```python
from build123d import *

# Parameters (mm, degrees)
ESQUISSE1_R             = 7
EXTRUSION1_DEPTH        = 100
ESQUISSE2_R             = 5
ESQUISSE2_R_2           = 2.5
EXTRUSION2_DEPTH        = 143
EXTRUSION2_DEPTH_BACK   = 36
ESQUISSE3_OUTSIDE_W     = 52.018
ESQUISSE3_OUTSIDE_H     = 52.018
ESQUISSE3_OUTSIDE_R     = 4.25
ENL_V_MAT_EXTRU_1_DEPTH = 3.5
ESQUISSE4_W             = 2
ESQUISSE4_H             = 3
ENL_V_MAT_EXTRU_2_DEPTH = 8
CHANFREIN1_SIZE         = 0.5


with BuildPart() as part:
    # Esquisse1 → Extrusion1 (new body)
    with BuildSketch(Plane(origin=(0, 0, 0), x_dir=(0, 0, -1), z_dir=(1, 0, 0))):
        Circle(ESQUISSE1_R)
    extrude(amount=EXTRUSION1_DEPTH)

    # Esquisse2 → Extrusion2 (add, two sides)
    with BuildSketch(Plane(origin=(0, 0, 0), x_dir=(0, 0, -1), z_dir=(1, 0, 0))) as extrusion2_sk:
        Circle(ESQUISSE2_R)
        Circle(ESQUISSE2_R_2, mode=Mode.SUBTRACT)
    extrude(amount=EXTRUSION2_DEPTH)
    extrude(extrusion2_sk.sketch, amount=-EXTRUSION2_DEPTH_BACK)

    # Esquisse3 outside → Enlèv. mat.-Extru.1 (cut)
    with BuildSketch(Plane.ZY.offset(36)):
        Rectangle(ESQUISSE3_OUTSIDE_W, ESQUISSE3_OUTSIDE_H)
        Circle(ESQUISSE3_OUTSIDE_R, mode=Mode.SUBTRACT)
    extrude(amount=-ENL_V_MAT_EXTRU_1_DEPTH, mode=Mode.SUBTRACT)

    # Esquisse4 → Enlèv. mat.-Extru.2 (cut, through all)
    with BuildSketch(Plane.XY):
        with Locations((-35, 0)):
            Rectangle(ESQUISSE4_W, ESQUISSE4_H)
    extrude(amount=ENL_V_MAT_EXTRU_2_DEPTH, mode=Mode.SUBTRACT)

    # Chanfrein1
    chanfrein1_edges = [part.edges().sort_by_distance(p)[0] for p in [
        (-36, 0, -4.25),
        (143, 0, 5),
    ]]
    chamfer(chanfrein1_edges, length=CHANFREIN1_SIZE)


solid = part.part
```
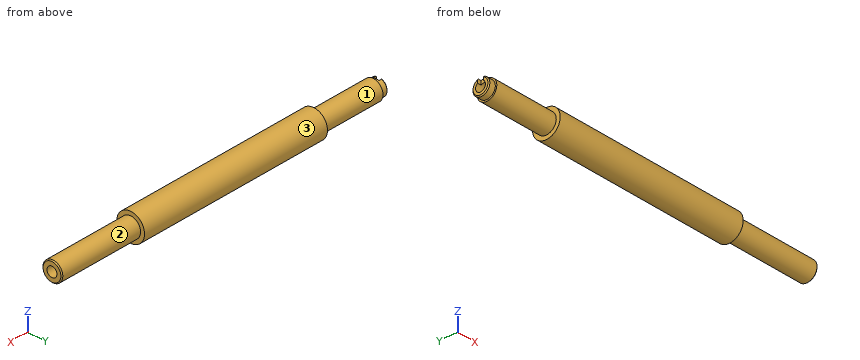
For this review, take the finished solid that the model builds, in its own axes (mm). Face numbers are marked on the shaded views. A direction names the side the tool comes from. Give positions to 0.01 mm unless a question says otherwise; leave off trailing zeros. Write each loop counter-clockwise with the first axis right and the second up, starting at its lowest first coordinate (ties: lowest second). Pieces come first, ordered by that corner, then holes.
Item 1: Wall thickness on probe 1 along Y at (x, z) = (-17.5, 0); probe 2 along X at (y, z) = (0.25, 2): over which ranges is each line inside the solid? List them lowest first.
Item 2: Take a section at B-B (z = 0). Give the boundary of the cut face in (x, y).
Item 3: Machinability: for the marked faces 1, 2 and 3, which of the approach directions +Z, -Z, +X, -X, +Y, -Y give a long, thin tool a straight path to every point of the face, cutting with its end or side? Answer none if there is none.
Item 4: Insertion check: P1, Ø5.5, axis at y = 1, z = -0.5, coming from the -X side; P2, Ø3, axis at x = 112, z = -1, coming from the -Y side; P3, Ø1, axis at x = 9, z = 5, coming from the -Y side; P4, Ø4, axis at x = 109, z = 4.5, coming from the -Y side. Each pin has a flat end and moves straight along its axis. Give the tip position at first contact, or say it passes through.
Item 5: Take a section at D-D (x = 60). Give the boundary of the cut face in (y, z).
Item 6: Take a section at A-A (y = 0). Give the boundary of the cut face in (x, z).
Item 7: Take a section at C-C (x = -16). Give the boundary of the cut face in (y, z).
Established:
1. probe 1: y = -5 to -2.5, 2.5 to 5
1. probe 2: x = 0 to 100
2. outline: (-36, -3.75) - (-35.5, -4.25) - (-32.5, -4.25) - (-32.5, -5) - (0, -5) - (0, -7) - (100, -7) - (100, -5) - (142.5, -5) - (143, -4.5) - (143, -2.5) - (100, -2.5) - (100, 2.5) - (143, 2.5) - (143, 4.5) - (142.5, 5) - (100, 5) - (100, 7) - (0, 7) - (0, 5) - (-32.5, 5) - (-32.5, 4.25) - (-35.5, 4.25) - (-36, 3.75) - (-36, 2.5) - (0, 2.5) - (0, -2.5) - (-36, -2.5) - close
3. face 1: -X
3. face 2: +X
3. face 3: +X, -X
4. P1: stops at x = -36
4. P2: stops at y = -5
4. P3: stops at y = -5.36
4. P4: stops at y = -4.33
5. outline: circle Ø14 at (0, 0)
6. outline: (-36, -3.75) - (-35.5, -4.25) - (-32.5, -4.25) - (-32.5, -5) - (0, -5) - (0, -7) - (100, -7) - (100, -5) - (142.5, -5) - (143, -4.5) - (143, -2.5) - (100, -2.5) - (100, 2.5) - (143, 2.5) - (143, 4.5) - (142.5, 5) - (100, 5) - (100, 7) - (0, 7) - (0, 5) - (-32.5, 5) - (-32.5, 4.25) - (-34, 4.25) - (-34, 2.5) - (0, 2.5) - (0, -2.5) - (-36, -2.5) - close
7. outline: circle Ø10 at (0, 0); hole circle Ø5 at (0, 0)
